Geometry: see drawing. Coordinates: mm, zero at the bounding-box minimum. A direction names the side the tool comes from. Coordinates: 2 decimals unless noted, no trailing zeros. Loops run counter-clockwise (first coordinate to the right, second up) from the corner with the lowest first, then second, coordinate; pieces in that order, holes last. Notation, with made-up numbers: (43, 52) - (78, 52) arc R35 cw to (78, 90) - close; hole circle Ø3 at (-18.75, 89). An arc over 180 degrees is marked (long way). Use a Markdown table: item, result. Add a question column.
1. Contact query for flat-ended pins moving along their axis: P1, Ø12, axis at x = 45, y = 10, coming from the +Z side; P2, Ø3, axis at y = 29, z = 3.5, coming from the +X side; P3, Ø3, axis at x = 29, z = 7, coming from the -Y side (1 decimal); P4, Ø4, axis at x = 47, z = 5, coming from the +Y side. Output: stop coordinate, or through.
2. Ray query, L1, parallel to Y at x = 5.5, z = 7.5; L2, parallel to Z at x = 3.5, y = 14.25; L3, parallel to X at y = 15.35, z = 5. Return the intervals inside material, ascending. Write a range as [from, to].
3. Section query D-D on x = 27. Return the cut outline in (y, z) (1 decimal).
4. Section query B-B on x = 3.5. Return the cut outline in (y, z), then the cut area to 3 significant figures.
5. Draft query along X for the marked faces 1, 2 and 3. Return one class per face: released by +X, released by -X, zero draft, split by the parting line, or undercut.
6. Section query C-C on y = 2.5. Return the cut outline in (x, z) (1 decimal).
7. Section query A-A on z = 5. State how many separate pieces and enclosed holes the cut face has, then the cut area to 3 significant figures.
8. Access query for the marked faces 4, 5, 6, 7 and 8. Directions: +Z, -Z, +X, -X, +Y, -Y. A direction counts if a zero-diameter tool reaches every point of the face in a straight line with its end or side. Return the directions, or none.
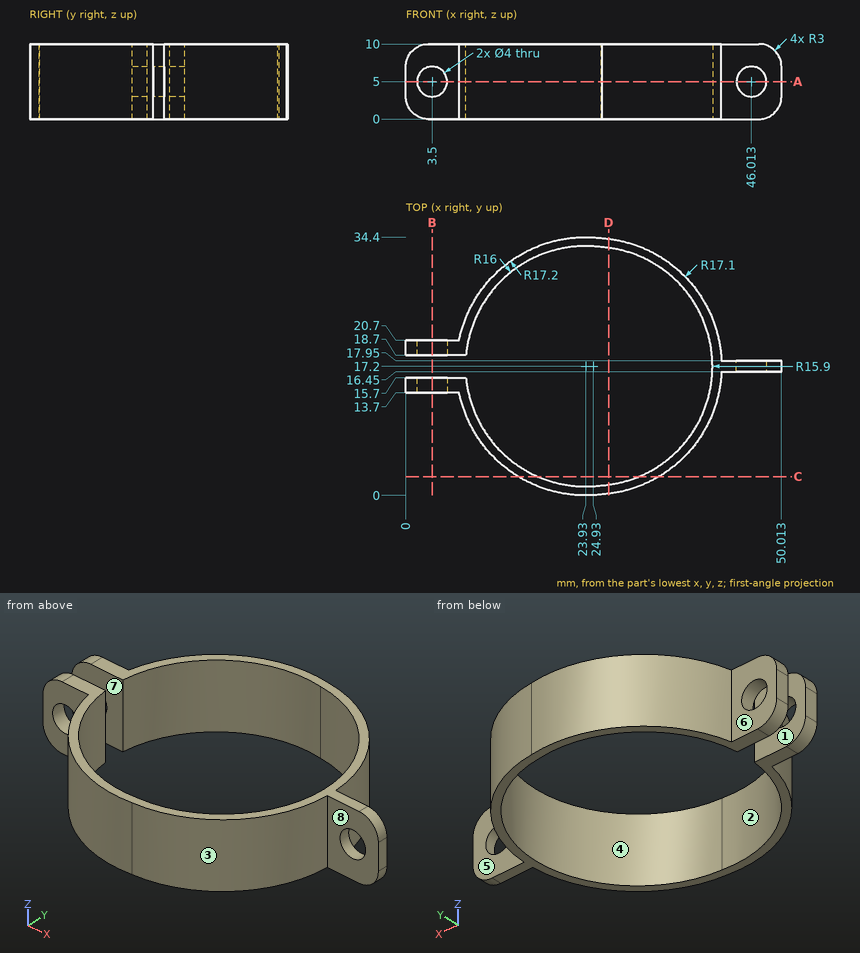
Resolved:
| question | item | result |
|---|---|---|
| 1 | P1 | z = 10 |
| 1 | P2 | x = 38.58 |
| 1 | P3 | y = 0.3 |
| 1 | P4 | y = 17.95 |
| 2 | L1 | [13.7, 15.7], [18.7, 20.7] |
| 2 | L2 | [0, 3], [7, 10] |
| 2 | L3 | [0, 1.5], [5.5, 8.04], [40.72, 41.93] |
| 3 | outline | (0.2, 0) - (1.4, 0) - (1.4, 10) - (0.2, 10) - close; (33, 0) - (34.2, 0) - (34.2, 10) - (33, 10) - close |
| 4 | outline | (13.7, 0) - (15.7, 0) - (15.7, 3) - (13.7, 3) - close; (13.7, 7) - (15.7, 7) - (15.7, 10) - (13.7, 10) - close; (18.7, 0) - (20.7, 0) - (20.7, 3) - (18.7, 3) - close; (18.7, 7) - (20.7, 7) - (20.7, 10) - (18.7, 10) - close |
| 4 | area | 24.0 mm² |
| 5 | face 1 | zero draft |
| 5 | face 2 | undercut |
| 5 | face 3 | released by +X |
| 6 | outline | (15, 0) - (17.6, 0) - (17.6, 10) - (15, 10) - close; (31, 0) - (33.7, 0) - (33.7, 10) - (31, 10) - close |
| 7 | separate pieces | 4 |
| 7 | enclosed holes | 0 |
| 7 | area | 141 mm² |
| 8 | face 4 | +Z, -Z |
| 8 | face 5 | +Z, -Z, +X, +Y |
| 8 | face 6 | +Z, -Z, -X, +Y |
| 8 | face 7 | +Z, -Z, -X |
| 8 | face 8 | +Z, -Z, +X, -Y |
